Can you work these out from the model? Positions are in its coordinate system, mm. A direction names the side the tool comes from. Give positions to 0.01 mm unless a question says otherwise; leave off trailing zeros. Write each loop counter-clockwise with the first axis right and the second up, starting at its lowest first coordinate (ties: lowest second). Pieces come first, ordered by that corner, then holes. Notation, with made-up numbers: M -5,-15 L 14,-15 A32 cw 14,22 Z; hole C 12.25,47.5 d9. An arc over 180 degrees is marked long. Use CSV: the item, a comma, the result in double quotes. Start each with the question number.
from build123d import *

# Parameters (mm, degrees)
CUT_EXTRUDE1_DEPTH      = 16.259152832
CUT_EXTRUDE1_DEPTH_BACK = 16.259152832
SKETCH2_R               = 1


with BuildPart() as part:
    # Sketch1 → Revolve1 (revolve)
    with BuildSketch(Plane.XY, mode=Mode.PRIVATE) as revolve1_sk:
        Polygon((0, 2.5), (0, 0), (8.84391273, 0), (14.84391273, 0), (14.84391273, 1.5), (6.84391273, 1.5), (6.84391273, 2.5), (5.1, 2.5), (5.1, 1.5), (3, 1.5), (3, 2.5), align=None)
    revolve(revolve1_sk.sketch.rotate(Axis((0, 0, 0), (1, 0, 0)), 180), axis=Axis((0, 0, 0), (1, 0, 0)))

    # Sketch2 → Cut-Extrude1 (cut, two sides: drawn at the far end of the back side and taken through both)
    with BuildSketch(Plane.XY.offset(-CUT_EXTRUDE1_DEPTH_BACK)):
        with Locations((12.84391273, 0)):
            Circle(SKETCH2_R)
    extrude(amount=CUT_EXTRUDE1_DEPTH + CUT_EXTRUDE1_DEPTH_BACK, mode=Mode.SUBTRACT)


solid = part.part
(1) I want a section at B-B (z = 0). Write out the boundary of the cut face in (x, y), and give its area (3 significant figures).
(2) Which directions (+Z, -Z, +X, -X, +Y, -Y) give clear straight access to the entire face, cutting with the end or side of a thin tool? Please do faces 5 (the face through (14.844, 0, 0)), 6 (the face through (5.1, -2, 0)), 7 (the face through (10.79, 1.11, -1.01)).
(3) I want a section at A-A (y = 0). Write out the boundary of the cut face in (x, z).
(4) Will these pins go through, and if not, where does the flat tip stop? pin 1 Ø2 at (x, z) = (10.5, -1.5) entering from -Y; pin 2 Ø1 at (x, z) = (12.5, 0) entering from +Y; pin 3 Ø3 at (x, z) = (8, -1) entering from -Y; pin 4 Ø1 at (x, y) = (5.5, 1) entering from -Z.
(5) I want a section at C-C (z = 1.15). Write out the boundary of the cut face in (x, y), and give its area (3 significant figures).
(6) I want a section at D-D (y = 1.2). Write out the boundary of the cut face in (x, z), and give its area (3 significant figures).
(7) Please list where these lines run through material, in increasing order: L1, parallel to X at y = 0, z = 0.65; L2, parallel to X at y = 0.75, z = 2.35; L3, parallel to Y at x = 8, z = 0.05. Write a range as [from, to].
(8) Thinking about a two-plate mould opening in X: for faces 1 (the face through (3, 0, 2)), 2 (the face through (6.844, 0, 2)), 3 (the face through (0, 0, 0)), 4 (the face through (12.05, -0.61, -0.02)), which applies, released by +X, released by -X, zero draft, split by the parting line, or undercut?
Geometry results:
1,outline,"M 0,-2.5 L 3,-2.5 L 3,-1.5 L 5.1,-1.5 L 5.1,-2.5 L 6.84,-2.5 L 6.84,-1.5 L 14.84,-1.5 L 14.84,1.5 L 6.84,1.5 L 6.84,2.5 L 5.1,2.5 L 5.1,1.5 L 3,1.5 L 3,2.5 L 0,2.5 Z; hole C 12.84,0 d2"
1,area,"50.9 mm2"
2,face 5,"+Z, -Z, +X, +Y, -Y"
2,face 6,"none"
2,face 7,"+X"
3,outline,"M 0,-2.5 L 3,-2.5 L 3,-1.5 L 5.1,-1.5 L 5.1,-2.5 L 6.84,-2.5 L 6.84,-1.5 L 11.84,-1.5 L 11.84,1.5 L 6.84,1.5 L 6.84,2.5 L 5.1,2.5 L 5.1,1.5 L 3,1.5 L 3,2.5 L 0,2.5 Z; M 13.84,-1.5 L 14.84,-1.5 L 14.84,1.5 L 13.84,1.5 Z"
4,pin 1,"stops at y = -1.41"
4,pin 2,"stops at y = 1.5"
4,pin 3,"stops at y = -2.5"
4,pin 4,"stops at z = -2.45"
5,outline,"M 0,-2.22 L 3,-2.22 L 3,-0.96 L 5.1,-0.96 L 5.1,-2.22 L 6.84,-2.22 L 6.84,-0.96 L 12.57,-0.96 A1 cw 12.57,0.96 L 6.84,0.96 L 6.84,2.22 L 5.1,2.22 L 5.1,0.96 L 3,0.96 L 3,2.22 L 0,2.22 Z; M 13.11,-0.96 L 14.84,-0.96 L 14.84,0.96 L 13.11,0.96 A1 cw Z"
5,area,"37.4 mm2"
6,outline,"M 0,-2.19 L 3,-2.19 L 3,-0.9 L 5.1,-0.9 L 5.1,-2.19 L 6.84,-2.19 L 6.84,-0.9 L 14.84,-0.9 L 14.84,0.9 L 6.84,0.9 L 6.84,2.19 L 5.1,2.19 L 5.1,0.9 L 3,0.9 L 3,2.19 L 0,2.19 Z"
6,area,"39.0 mm2"
7,L1,"x = [0, 11.84], [13.84, 14.84]"
7,L2,"x = [0, 3], [5.1, 6.84]"
7,L3,"y = [-1.5, 1.5]"
8,face 1,"undercut"
8,face 2,"released by +X"
8,face 3,"released by -X"
8,face 4,"undercut"
